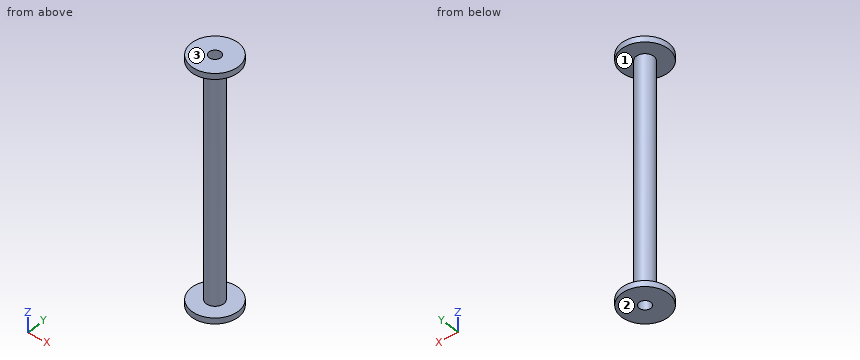
from build123d import *

# Parameters (mm, degrees)
SKETCH1_R           = 19.05
SKETCH1_R_2         = 12.7
BOSS_EXTRUDE1_DEPTH = 266.7
BOSS_EXTRUDE2_START = -12.7
SKETCH2_R           = 50.8
SKETCH2_R_2         = 12.7
BOSS_EXTRUDE2_DEPTH = 12.7
SKETCH3_R           = 50.8
SKETCH3_R_2         = 12.7
BOSS_EXTRUDE3_DEPTH = 12.7


with BuildPart() as part:
    # Sketch1 → Boss-Extrude1 (new, symmetric)
    with BuildSketch(Plane.XY):
        Circle(SKETCH1_R)
        Circle(SKETCH1_R_2, mode=Mode.SUBTRACT)
    extrude(amount=BOSS_EXTRUDE1_DEPTH, both=True)

    # Sketch2 → Boss-Extrude2 (add)
    with BuildSketch(Plane.XY.offset(266.7).offset(BOSS_EXTRUDE2_START)):
        Circle(SKETCH2_R)
        Circle(SKETCH2_R_2, mode=Mode.SUBTRACT)
    extrude(amount=BOSS_EXTRUDE2_DEPTH)

    # Sketch3 → Boss-Extrude3 (add)
    with BuildSketch(Plane(origin=(0, 0, -266.7), x_dir=(-1, 0, 0), z_dir=(0, 0, -1))):
        with Locations(Location((0, 0, 0), (0, 0, 180))):
            Circle(SKETCH3_R)
        with Locations(Location((0, 0, 0), (0, 0, 180))):
            Circle(SKETCH3_R_2, mode=Mode.SUBTRACT)
    extrude(amount=-BOSS_EXTRUDE3_DEPTH)


solid = part.part
CAD build for the part. Positions are in the model's coordinates, mm. Face numbers are marked on the shaded views. Give positions to 0.01 mm unless a question says otherwise; leave off trailing zeros. Loops run counter-clockwise (first coordinate to the right, second up) from the corner with the lowest first, then second, coordinate; pieces in that order, holes last. Notation, with made-up numbers: M 20.5,-26.5 L 76.5,-26.5 A28 cw 76.5,10.5 Z; hole C -16.75,50.25 d7. An arc over 180 degrees is marked long. One line per question, with ' | ' between items. Start each with the question number.
1. Probe L1, parallel to Z at x = 18, y = -24.5; L2, parallel to Y at x = 11, z = 198; L3, parallel to X at y = 4.5, z = -180. List the from-to ranges inside material, lowest first. Write a range as from..to.
2. Saw through at D-D on x = -33. Give the cut face in (y, z).
3. Two-plate mould, pull along Z, no slides. Class the marked faces 1, 2 and 3: pulls with the +Z half, pulls with the -Z half, needs draft (parallel to the pull), parting line crosses it, or undercut.
4. Flat gauge pins, fed straight in: pin 1 (10 mm diameter, centred on y = -16, z = 137.5, fed in from -X); pin 2 (2 mm diameter, centred on y = -1, z = -183.5, fed in from +X). Where does each tip first touch, or does it go through?
5. Saw through at A-A on x = 0. Give the cut face in (y, z).
6. Saw through at C-C on z = 114.5. Give the cut face in (x, y), plus the area to 3 significant figures.
Result sheet:
1) L1: z = -266.7..-254, 254..266.7 | L2: y = -15.55..-6.35, 6.35..15.55 | L3: x = -18.51..-11.88, 11.88..18.51
2) outline: M -38.62,-266.7 L 38.62,-266.7 L 38.62,-254 L -38.62,-254 Z; M -38.62,254 L 38.62,254 L 38.62,266.7 L -38.62,266.7 Z
3) face 1: undercut | face 2: pulls with the -Z half | face 3: pulls with the +Z half
4) pin 1: stops at x = -15.55 | pin 2: stops at x = 19.05
5) outline: M -50.8,-266.7 L -12.7,-266.7 L -12.7,266.7 L -50.8,266.7 L -50.8,254 L -19.05,254 L -19.05,-254 L -50.8,-254 Z; M 12.7,-266.7 L 50.8,-266.7 L 50.8,-254 L 19.05,-254 L 19.05,254 L 50.8,254 L 50.8,266.7 L 12.7,266.7 Z
6) outline: C 0,0 d38.1; hole C 0,0 d25.4 | area: 633 mm^2
